Autodesk Inventor part; units mm, degrees
ref_plane "Work Plane1" through (-29.1, -14.5, 2.4) normal (0, 0, -1) x (0, 1, 0)
ref_plane "Work Plane2" through (-13.8999, -10.5497, 2.25) normal (0, 0, -1) x (0, 1, 0)
ref_plane "Work Plane4" through (-16.9391, -17.02, 0.2169) normal (0, 0, 1) x (1, 0, 0)
ref_plane "Work Plane1" through (-29.1, -14.5, 2.4) normal (0, 0, -1) x (0, 1, 0)
ref_plane "Work Plane2" through (-13.8999, -10.5497, 2.25) normal (0, 0, -1) x (0, 1, 0)
sketch "Sketch1" plane through (0, 0, 0) normal (0, 0, 1) x (1, 0, 0)
  line L0 (-34.86, 0) -> (34.86, 0) construction
  line L1 (0, -34.86) -> (0, 34.86) construction
  line L2 (0, 0) -> (11.1575, 11.1575) construction
  line L3 (0, 0) -> (15.7791, 0) construction
  line L4 (0, 24.9) -> (16.8009, 24.9)
  line L5 (16.8009, 24.9) -> (16.8009, 21.2415)
  line L6 (16.8009, 21.2415) -> (19.0212, 19.0212)
  line L7 (24.9, 0) -> (24.9, 16.8009)
  line L8 (24.9, 16.8009) -> (21.2415, 16.8009)
  line L9 (21.2415, 16.8009) -> (19.0212, 19.0212)
  line L10 (0, -24.9) -> (16.8009, -24.9)
  line L11 (16.8009, -24.9) -> (16.8009, -21.2415)
  line L12 (16.8009, -21.2415) -> (19.0212, -19.0212)
  line L13 (24.9, 0) -> (24.9, -16.8009)
  line L14 (24.9, -16.8009) -> (21.2415, -16.8009)
  line L15 (21.2415, -16.8009) -> (19.0212, -19.0212)
  line L16 (0, 24.9) -> (-16.8009, 24.9)
  line L17 (-16.8009, 24.9) -> (-16.8009, 21.2415)
  line L18 (-16.8009, 21.2415) -> (-19.0212, 19.0212)
  line L19 (-24.9, 16.8009) -> (-21.2415, 16.8009)
  line L20 (-21.2415, 16.8009) -> (-19.0212, 19.0212)
  line L21 (0, -24.9) -> (-16.8009, -24.9)
  line L22 (-16.8009, -24.9) -> (-16.8009, -21.2415)
  line L23 (-16.8009, -21.2415) -> (-19.0212, -19.0212)
  line L24 (-21.2415, -16.8009) -> (-19.0212, -19.0212)
  line L25 (-24.9, -16.8009) -> (-21.2415, -16.8009)
  line L26 (-24.9, 0) -> (-24.9, -16.8009)
  line L27 (-24.9, 0) -> (-24.9, 16.8009)
  circle A0 centre (0, 0) radius 3
  dimension "d0" = 45
  dimension "d2" = 24.9
  dimension "d3" = 3.14
  dimension "d4" = 26.9
  dimension "d5" = 6
extrude "Extrusion1" add sketch "Sketch1" along normal blind 6
ref_plane "Work Plane4" through (-16.9391, -17.02, 0.2169) normal (0, 0, 1) x (1, 0, 0)
sketch "Skizze6" plane through (-16.8009, 24.9, 6) normal (0, 0, 1) x (1, 0, 0)
  circle A0 centre (6.8009, -18) radius 1.65 construction
  circle A1 centre (3.0009, -24.9) radius 1.65 construction
  circle A2 centre (26.5009, -34.9) radius 1.65 construction
  circle A3 centre (26.5009, -14.9) radius 1.65 construction
  circle A4 centre (16.8009, -24.9) radius 10 construction
  line L0 (33.6017, -3.6585) -> (33.6017, 0)
  line L1 (33.6017, 0) -> (0, 0) construction
  line L2 (0, 0) -> (0, -3.6585)
  line L3 (0, -3.6585) -> (-4.4406, -8.0991)
  line L4 (-4.4406, -8.0991) -> (-8.0991, -8.0991)
  line L5 (-8.0991, -8.0991) -> (-8.0991, -41.7009) construction
  line L6 (-8.0991, -41.7009) -> (-4.4406, -41.7009)
  line L7 (-4.4406, -41.7009) -> (0, -46.1415)
  line L8 (0, -46.1415) -> (0, -49.8)
  line L9 (0, -49.8) -> (33.6017, -49.8) construction
  line L10 (33.6017, -49.8) -> (33.6017, -46.1415)
  line L11 (33.6017, -46.1415) -> (38.0423, -41.7009)
  line L12 (38.0423, -41.7009) -> (41.7009, -41.7009)
  line L13 (41.7009, -41.7009) -> (41.7009, -8.0991) construction
  line L14 (41.7009, -8.0991) -> (38.0423, -8.0991)
  line L15 (38.0423, -8.0991) -> (33.6017, -3.6585)
  line L16 (-0.2, 0.2) -> (33.8017, 0.2) construction
  line L17 (33.8017, 0.2) -> (33.8017, -3.5757)
  line L18 (33.8017, -3.5757) -> (38.1252, -7.8991)
  line L19 (38.1252, -7.8991) -> (41.9009, -7.8991)
  line L20 (41.9009, -7.8991) -> (41.9009, -41.9009) construction
  line L21 (41.9009, -41.9009) -> (38.1252, -41.9009)
  line L22 (38.1252, -41.9009) -> (33.8017, -46.2243)
  line L23 (33.8017, -46.2243) -> (33.8017, -50)
  line L24 (33.8017, -50) -> (-0.2, -50) construction
  line L25 (-0.2, -50) -> (-0.2, -46.2243)
  line L26 (-0.2, -46.2243) -> (-4.5235, -41.9009)
  line L27 (-4.5235, -41.9009) -> (-8.2991, -41.9009)
  line L28 (-8.2991, -41.9009) -> (-8.2991, -7.8991) construction
  line L29 (-8.2991, -7.8991) -> (-4.5235, -7.8991)
  line L30 (-4.5235, -7.8991) -> (-0.2, -3.5757)
  line L31 (-0.2, -3.5757) -> (-0.2, 0.2)
  line L32 (-8.0991, -8.0991) -> (-8.0991, -7.8991)
  line L33 (0, 0) -> (-0.2, 0)
  line L34 (33.6017, 0) -> (33.8017, 0)
  line L35 (41.7009, -8.0991) -> (38.0423, -8.0991)
  line L36 (41.7009, -8.0991) -> (41.7009, -7.8991)
  line L37 (41.7009, -41.7009) -> (41.7009, -41.9009)
  line L38 (33.6017, -49.8) -> (33.8017, -49.8)
  line L39 (-8.0991, -41.7009) -> (-8.0991, -41.9009)
  line L40 (0, -49.8) -> (-0.2, -49.8)
  point P0 (16.8009, -24.9)
  dimension "d25" = 0.2
extrude "IM_offset" add sketch "Skizze6" against normal up to surface (5.7831 mm away)
ref_plane "Work Plane3" through (-17.0009, 0, 0) normal (0, -1, 0) x (1, 0, 0)
sketch "Sketch7" plane through (-17.0009, 0, 0) normal (0, -1, 0) x (1, 0, 0)
  line L0 (6.6601, 19.3407) -> (38.4799, -12.4791)
  line L1 (38.4799, -12.4791) -> (32.4799, -18.4791)
  line L2 (32.4799, -18.4791) -> (0.6601, 13.3407)
  line L3 (0.6601, 13.3407) -> (6.6601, 19.3407)
  line L4 (6.6601, 19.3407) -> (51.6601, 19.3407) construction
  line L5 (14.0009, 6) -> (20.0009, 6)
  line L6 (20.0009, 0) -> (14.0009, 0)
  point P0 (17.0009, 0)
  dimension "d28" = 45
  dimension "d29" = 45
extrude "Extrusion6" cut sketch "Sketch7" along normal mid plane 30
sketch "Sketch8" plane through (24.9, 16.8009, 6) normal (1, 0, 0) x (0, 0, -1)
  line L0 (6, 0) -> (6, -33.6017)
  line L1 (0, -33.8017) -> (0, 0.2)
  line L2 (0, -33.8017) -> (5.7831, -33.8017)
  circle A0 centre (0, -16.8009) radius 5
  line L3 (0, 0.2) -> (5.7831, 0.2)
  line L4 (6, 0) -> (5.7831, 0)
  line L5 (5.7831, 0.2) -> (5.7831, 0)
  line L6 (5.7831, -33.6017) -> (5.7831, -33.8017)
  line L7 (6, -33.6017) -> (5.7831, -33.6017)
  point P0 (6, -16.8009)
  dimension "d32" = 10
extrude "Extrusion7" cut sketch "Sketch8" against normal blind 30 contours A0 L1 | L1 A0
fillet "Fillet1" radius 4 2 edges at (13.95, 5, 6) (13.95, -5, 6)
properties part number "20_Cube_insert_Fluorescence_Darkfield_Mirror_v3"
Can you work these out from the model? Positions are in its coordinate system, mm. A direction names the side the tool comes from. Give positions to 0.01 mm unless a question says otherwise; leave off trailing zeros. Order: outer loops, then holes, each group sorted by start corner. A loop starts at its lowest first (then second) coordinate and runs counter-clockwise, first axis right, second up. Notation, with made-up numbers: (-35.75, 46) - (6.25, 46) arc R20 cw to (6.25, 82) - close; hole circle Ø1 at (29, -0.5). An arc over 180 degrees is marked (long way). Use a Markdown table: item, result. Add a question column.
Q1. Please list where these lines run through material, in increasing order: line 1 along Y through (x, z) = (-3, 1.75); line 2 along X through (y, z) = (2, 1.25); line 3 along Y through (x, z) = (14.5, 5).
Q2. If we section it at B-B on y = 13: Write out the boundary of the cut face in (x, z), plus the area to 3 significant figures.
Q3. If we section it at D-D on z = 4.5: Write out the boundary of the cut face in (x, y).
Q4. If we section it at C-C on x = -6: Write out the boundary of the cut face in (y, z), plus the area to 3 significant figures.
Q5. If we section it at A-A on x = -1: Write out the boundary of the cut face in (y, z).
Q6. I'm going to push flat-ended pins straight in: pin 1 (1.1 mm diameter, centred on y = 23.5, z = 3, fed in from -X); pin 2 (3 mm diameter, centred on y = -23, z = 3, fed in from +X); pin 3 (1.1 mm diameter, centred on x = 23.5, z = 4.5, fed in from -Y). Where does each tip first touch, or does it pass through?
Q7. If we mould it in two halves opening along X, with no side actions, what happens to faces 4 (the flat face through (-5.1, 0, 1.7)), 5 (the flat face through (-17.001, 23, 3)), 6 (the flat face through (0, -15, 3))? For each: released by +X, released by -X, zero draft, split by the parting line, or undercut.
Q8. On a 3-axis mill with a long thin cutter (end or side, diameter ignored), from which of +Z, -Z, +X, -X, +Y, -Y can I reach the whole of each face in a straight line? I mean faces 1 (the cylindrical face through (14.103, 5.981, 5.416)), 2 (the flat face through (17.001, 23, 3)), 3 (the flat face through (-23, -17.001, 3)). Say none if no direction works.
Answers follow:
| question | item | result |
|---|---|---|
| 1 | line 1 | y = -24.9 to -15, 15 to 24.9 |
| 1 | line 2 | x = -24.9 to -4.25, 7.75 to 24.9 |
| 1 | line 3 | y = -24.9 to -5.42, 5.42 to 24.9 |
| 2 | outline | (-24.9, 0) - (-3, 0) - (-9, 6) - (-24.9, 6) - close; (3, 6) - (9, 0) - (24.9, 0) - (24.9, 6) - close |
| 2 | area | 227 mm^2 |
| 3 | outline | (-24.9, -17) - (-21.32, -17) - (-17, -21.32) - (-17, -24.9) - (17, -24.9) - (17, -21.32) - (21.32, -17) - (24.9, -17) - (24.9, -4.94) - (4.5, -4.94) - (4.5, -15) - (-7.5, -15) - (-7.5, 15) - (4.5, 15) - (4.5, 4.94) - (24.9, 4.94) - (24.9, 17) - (21.32, 17) - (17, 21.32) - (17, 24.9) - (-17, 24.9) - (-17, 21.32) - (-21.32, 17) - (-24.9, 17) - close |
| 4 | outline | (-24.9, 0) - (24.9, 0) - (24.9, 6) - (15, 6) - (15, 3) - (-15, 3) - (-15, 6) - (-24.9, 6) - close |
| 4 | area | 209 mm^2 |
| 5 | outline | (-24.9, 0) - (-15, 0) - (-15, 6) - (-24.9, 6) - close; (15, 0) - (24.9, 0) - (24.9, 6) - (15, 6) - close |
| 6 | pin 1 | stops at x = -17 |
| 6 | pin 2 | stops at x = 17 |
| 6 | pin 3 | stops at y = -17 |
| 7 | face 4 | released by +X |
| 7 | face 5 | released by -X |
| 7 | face 6 | undercut |
| 8 | face 1 | +Z, +X |
| 8 | face 2 | +Z, -Z, +X, +Y |
| 8 | face 3 | +Z, -Z, -X, -Y |
